Source: CAD feature listing. Evaluate the final solid. Frame: model axes, mm. Face numbers are marked on the shaded views. Give positions to 0.01 mm unless a question says otherwise; leave off trailing zeros. Loops run counter-clockwise (first coordinate to the right, second up) from the corner with the lowest first, then second, coordinate; pieces in that order, holes last. Notation, with made-up numbers: (-26.5, 1.25) -> (20.5, 1.25) arc R23 ccw to (20.5, 39.25) -> close; hole circle Ø8 at (63, -9.75). An arc over 180 degrees is marked (long way). Return JSON: item names as keys, results as strings. Group by question number.
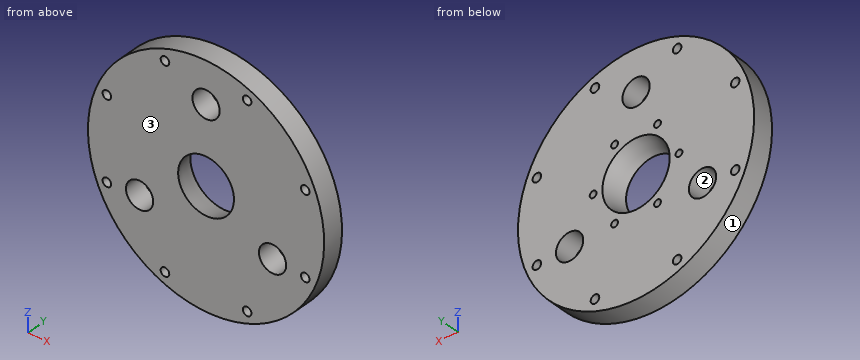
```python
from build123d import *

# Parameters (mm, degrees)
SKETCH1_R           = 55
BOSS_EXTRUDE1_DEPTH = 10
SKETCH6_R           = 2
CUT_EXTRUDE3_DEPTH  = 79.421935707
CIRPATTERN1_COUNT   = 8
SKETCH7_R           = 6.35
CUT_EXTRUDE4_DEPTH  = 79.421935707
CIRPATTERN2_COUNT   = 3
SKETCH8_R           = 1.5875
CUT_EXTRUDE5_DEPTH  = 7
CIRPATTERN3_COUNT   = 6


with BuildPart() as part:
    # Sketch1 → Boss-Extrude1 (new body)
    with BuildSketch(Plane(origin=(0, 0, 0), x_dir=(1, 0, 0), z_dir=(0, 1, 0))):
        with Locations(Location((0, 0, 0), (0, 0, 270))):
            Circle(SKETCH1_R)
    extrude(amount=BOSS_EXTRUDE1_DEPTH)

    # Sketch5 → Cut-Revolve1 (revolve, cut)
    with BuildSketch(Plane.XY, mode=Mode.PRIVATE) as cut_revolve1_sk:
        Polygon((0, 0), (0, 10), (15.679491924, 10), (13, 0), align=None)
    revolve(cut_revolve1_sk.sketch.rotate(Axis((0, 0, 0), (0, 1, 0)), 90), axis=Axis((0, 0, 0), (0, 1, 0)), mode=Mode.SUBTRACT)

    # Sketch6 → Cut-Extrude3 (cut, through all)
    with BuildSketch(Plane(origin=(0, 0, 0), x_dir=(1, 0, 0), z_dir=(0, 1, 0))):
        with Locations(Location((46.193976626, 19.134171618, 0), (0, 0, 270))):
            Circle(SKETCH6_R)
    cut_extrude3 = extrude(amount=CUT_EXTRUDE3_DEPTH, mode=Mode.SUBTRACT)

    # CirPattern1: Cut-Extrude3 ×8 about axis
    cirpattern1_axis = Axis((0, 0, 0), (0, 1, 0))
    for i in range(1, CIRPATTERN1_COUNT):
        add(cut_extrude3.rotate(cirpattern1_axis, i * 360 / CIRPATTERN1_COUNT), mode=Mode.SUBTRACT)

    # Sketch7 → Cut-Extrude4 (cut, through all)
    with BuildSketch(Plane(origin=(0, 10, 0), x_dir=(1, 0, 0), z_dir=(0, 1, 0))):
        with Locations(Location((30.960408185, 17.875, 0), (0, 0, 270))):
            Circle(SKETCH7_R)
    cut_extrude4 = extrude(amount=-CUT_EXTRUDE4_DEPTH, mode=Mode.SUBTRACT)

    # CirPattern2: Cut-Extrude4 ×3 about axis
    cirpattern2_axis = Axis((0, 0, 0), (0, 1, 0))
    for i in range(1, CIRPATTERN2_COUNT):
        add(cut_extrude4.rotate(cirpattern2_axis, i * 360 / CIRPATTERN2_COUNT), mode=Mode.SUBTRACT)

    # Sketch8 → Cut-Extrude5 (cut)
    with BuildSketch(Plane(origin=(0, 10, 0), x_dir=(1, 0, 0), z_dir=(0, 1, 0))):
        with Locations(Location((20, 0, 0), (0, 0, 270))):
            Circle(SKETCH8_R)
    cut_extrude5 = extrude(amount=-CUT_EXTRUDE5_DEPTH, mode=Mode.SUBTRACT)

    # CirPattern3: Cut-Extrude5 ×6 about axis
    cirpattern3_axis = Axis((0, 0, 0), (0, 1, 0))
    for i in range(1, CIRPATTERN3_COUNT):
        add(cut_extrude5.rotate(cirpattern3_axis, i * 360 / CIRPATTERN3_COUNT), mode=Mode.SUBTRACT)


solid = part.part
```
1) Cut plane C-C on z = 35.75. Return loops of the section in (x, y), then the cut area to 3 significant figures.
2) Cut plane D-D on x = 41. Return loops of the section in (y, z), then the cut area to 3 significant figures.
3) Mould query, pull axis X, two halves, no side actions, for the marked faces 1, 2 and 3. Classes: released by +X, released by -X, zero draft, split by the parting line, or undercut.
4) Material intervals for line 1 (Z direction, x = 45.5, y = 7.5); line 2 (Z direction, x = -20, y = 9.75); line 3 (Z direction, x = -5.5, y = 2.5), sorted ascending.
5) Contact query for flat-ended pins moving along their axis: P1, Ø5, axis at x = 46.19, z = 19.13, coming from the +Y side; P2, Ø1.5, axis at x = -32.5, y = 4, coming from the -Z side; P3, Ø4, axis at y = 4.5, z = -6.5, coming from the +X side; P4, Ø1, axis at x = -10.5, z = -17.5, coming from the +Y side. Output: stop coordinate, or through.
6) Cut plane A-A on x = 0. Return loops of the section in (y, z), then the cut area to 3 significant figures.
7) Cut plane B-B on y = 4.25. Count the separate pieces of the cut face and the enclosed holes in it, then the cut area to 3 significant figures.
Calculated:
{
 "1": {"outline": "(-41.8, 0) -> (-6.35, 0) -> (-6.35, 10) -> (-41.8, 10) -> close; (6.35, 0) -> (41.8, 0) -> (41.8, 10) -> (6.35, 10) -> close", "area": "709 mm2"},
 "2": {"outline": "(0, -36.66) -> (10, -36.66) -> (10, 36.66) -> (0, 36.66) -> close", "area": "733 mm2"},
 "3": {"face 1": "split by the parting line", "face 2": "undercut", "face 3": "zero draft"},
 "4": {"line 1": "-30.9 to -21.01, -17.26 to 17.26, 21.01 to 30.9", "line 2": "-51.23 to -48, -44.39 to -1.59, 1.59 to 44.39, 48 to 51.23", "line 3": "-54.72 to -12.51, 12.51 to 32.58, 38.92 to 54.72"},
 "5": {"P1": "y = 10", "P2": "z = -44.91", "P3": "x = 54.82", "P4": "y = 3"},
 "6": {"outline": "(0, -55) -> (10, -55) -> (10, -15.68) -> (0, -13) -> close; (0, 13) -> (10, 15.68) -> (10, 29.4) -> (0, 29.4) -> close; (0, 42.1) -> (10, 42.1) -> (10, 55) -> (0, 55) -> close", "area": "686 mm2"},
 "7": {"separate pieces": "1", "enclosed holes": "18", "area": "8,350 mm2"}
}
